Build history of the part. All positions in model axes, mm. Face numbers are marked on the shaded views. A direction names the side the tool comes from. Round coordinates to 2 decimals unless told otherwise and drop trailing zeros. Order: outer loops, then holes, each group sorted by start corner. A loop starts at its lowest first (then second) coordinate and runs counter-clockwise, first axis right, second up. Notation, with made-up numbers: (14, 10.5) -> (41, 10.5) arc R24 ccw to (41, 22.5) -> close; hole circle Ø2 at (61, 23). An arc over 180 degrees is marked (long way). Use a Markdown table: item, result. Add a question column.
Item 1: Slice it at A-A, the plane x = 0. Give the cut face in (y, z).
Item 2: Probe L1, parallel to X at y = -1.75, z = 0.5; L2, parallel to X at y = 2, z = 1.75; L3, parallel to Y at x = 0, z = 1.45. List the from-to ranges inside material, lowest first.
Item 3: Slice it at D-D, the plane x = -5. Give the cut face in (y, z).
Item 4: Slice it at C-C, the plane z = 3.6. Give the cut face in (x, y), plus the area to 3 significant figures.
Item 5: 3-axis set-ups, long thin cutter, end or side, ignore diameter. For the marked faces 1, 2 and 3: which of +Z, -Z, +X, -X, +Y, -Y reach the whole face in a straight line?
Item 6: Pin check, flat tips, straight feed: pin 1 (1.5 mm diameter, centred on x = 4, y = -1.5, fed in from +Z); pin 2 (2 mm diameter, centred on x = -5, z = 0.5, fed in from +Y); pin 3 (2 mm diameter, centred on y = -4.5, z = 1, fed in from -X). Stop position of each tip, or through.
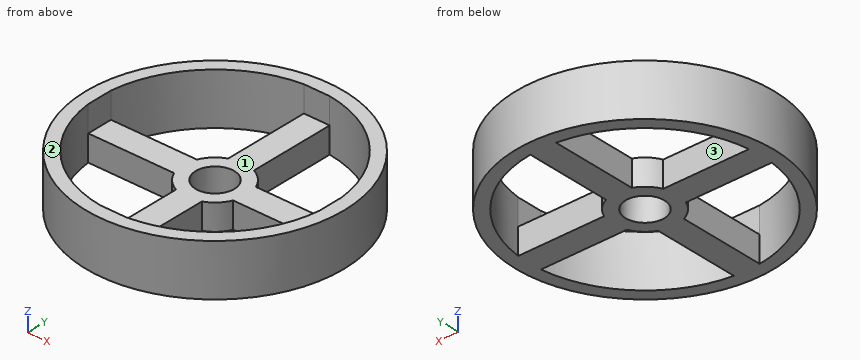
from build123d import *

# Parameters (mm, degrees)
F0_R     = 1.5
F1_DEPTH = 2
F0_R_2   = 10
F2_DEPTH = 4


with BuildPart() as f1:
    # F0 (on Top) → F1 (new body)
    with BuildSketch(Plane.XY):
        with BuildLine():
            Line((-8.944272, 1), (-8.944272, -1))
            Line((-8.944272, -1), (-2.291288, -1))
            ThreePointArc((-2.291288, -1), (-1.767767, -1.767767), (-1, -2.291288))
            Line((-1, -2.291288), (-1, -8.944272))
            Line((-1, -8.944272), (1, -8.944272))
            Line((1, -8.944272), (1, -2.291288))
            ThreePointArc((1, -2.291288), (1.767767, -1.767767), (2.291288, -1))
            Line((2.291288, -1), (8.944272, -1))
            Line((8.944272, -1), (8.944272, 1))
            Line((8.944272, 1), (2.291288, 1))
            ThreePointArc((2.291288, 1), (1.767767, 1.767767), (1, 2.291288))
            Line((1, 2.291288), (1, 8.944272))
            Line((1, 8.944272), (-1, 8.944272))
            Line((-1, 8.944272), (-1, 2.291288))
            ThreePointArc((-1, 2.291288), (-1.767767, 1.767767), (-2.291288, 1))
            Line((-2.291288, 1), (-8.944272, 1))
        make_face()
        Circle(F0_R, mode=Mode.SUBTRACT)
    extrude(amount=F1_DEPTH)

    # F0 (on Top) → F2 (join)
    with BuildSketch(Plane.XY):
        Circle(F0_R_2)
        with BuildLine():
            ThreePointArc((-1, -8.944272), (-6.363961, -6.363961), (-8.944272, -1))
            Line((-8.944272, -1), (-8.944272, 1))
            ThreePointArc((-8.944272, 1), (-6.363961, 6.363961), (-1, 8.944272))
            Line((-1, 8.944272), (1, 8.944272))
            ThreePointArc((1, 8.944272), (6.363961, 6.363961), (8.944272, 1))
            Line((8.944272, 1), (8.944272, -1))
            ThreePointArc((8.944272, -1), (6.363961, -6.363961), (1, -8.944272))
            Line((1, -8.944272), (-1, -8.944272))
        make_face(mode=Mode.SUBTRACT)
    extrude(amount=F2_DEPTH)


solid = f1.part
Check sheet entries:
| question | item | result |
|---|---|---|
| 1 | outline | (-10, 0) -> (-1.5, 0) -> (-1.5, 2) -> (-8.94, 2) -> (-8.94, 4) -> (-10, 4) -> close; (1.5, 0) -> (10, 0) -> (10, 4) -> (8.94, 4) -> (8.94, 2) -> (1.5, 2) -> close |
| 2 | L1 | -9.85 to -8.83, -1.79 to 1.79, 8.83 to 9.85 |
| 2 | L2 | -9.8 to -8.77, -1.5 to 1.5, 8.77 to 9.8 |
| 2 | L3 | -10 to -1.5, 1.5 to 10 |
| 3 | outline | (-8.66, 0) -> (-7.48, 0) -> (-7.48, 4) -> (-8.66, 4) -> close; (-1, 0) -> (1, 0) -> (1, 2) -> (-1, 2) -> close; (7.48, 0) -> (8.66, 0) -> (8.66, 4) -> (7.48, 4) -> close |
| 4 | outline | circle Ø20 at (0, 0); hole (-8.94, -1) arc R9 ccw to (-1, -8.94) -> (1, -8.94) arc R9 ccw to (8.94, -1) -> (8.94, 1) arc R9 ccw to (1, 8.94) -> (-1, 8.94) arc R9 ccw to (-8.94, 1) -> close |
| 4 | area | 60.0 mm2 |
| 5 | face 1 | +Z |
| 5 | face 2 | +Z, +X, -X, +Y, -Y |
| 5 | face 3 | +Z, -Z |
| 6 | pin 1 | z = 2 |
| 6 | pin 2 | y = 9.17 |
| 6 | pin 3 | x = -9.37 |
